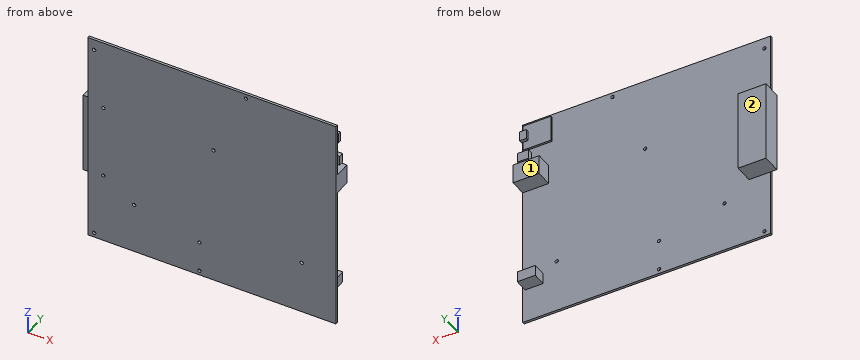
from build123d import *

# Parameters (mm, degrees)
SKETCH1_W               = 203.2
SKETCH1_H               = 177.8
BOSS_EXTRUDE1_DEPTH     = 2
SKETCH3_W               = 21.35
SKETCH3_H               = 16
BOSS_EXTRUDE2_DEPTH     = 13.4
CUT_EXTRUDE1_DEPTH      = 136.666244881
CUT_EXTRUDE1_DEPTH_BACK = 136.666244881
SKETCH2_R               = 1.397
SKETCH4_W               = 22.86
SKETCH4_H               = 67.056
BOSS_EXTRUDE3_DEPTH     = 15.24
SKETCH5_W               = 14.75
SKETCH5_H               = 8.9
BOSS_EXTRUDE4_DEPTH     = 10.922
SKETCH7_W               = 9
SKETCH7_H               = 7.75
BOSS_EXTRUDE5_DEPTH     = 4
SKETCH8_W               = 22.9
SKETCH8_H               = 21.57
BOSS_EXTRUDE6_DEPTH     = 1.6
SKETCH9_W               = 5.5
SKETCH9_H               = 8
BOSS_EXTRUDE7_DEPTH     = 2.7


with BuildPart() as part:
    # Sketch1 → Boss-Extrude1 (new body)
    with BuildSketch(Plane(origin=(0, 0, 0), x_dir=(1, 0, 0), z_dir=(0, 1, 0))):
        Rectangle(SKETCH1_W, SKETCH1_H)
    extrude(amount=BOSS_EXTRUDE1_DEPTH)

    # Sketch3 → Boss-Extrude2 (add)
    with BuildSketch(Plane(origin=(0, 2, 0), x_dir=(1, 0, 0), z_dir=(0, 1, 0))):
        with Locations((90.925, -35.94)):
            Rectangle(SKETCH3_W, SKETCH3_H)
    extrude(amount=BOSS_EXTRUDE2_DEPTH)

    # Sketch2 → Cut-Extrude1 (cut, two sides: drawn at the far end of the back side and taken through both)
    with BuildSketch(Plane(origin=(0, 2, 0), x_dir=(1, 0, 0), z_dir=(0, 1, 0)).offset(-CUT_EXTRUDE1_DEPTH_BACK)):
        with Locations(Location((-96.52, 85.09, 0), (0, 0, 270))):
            Circle(SKETCH2_R)
        with Locations(Location((-10.16, 85.09, 0), (0, 0, 270))):
            Circle(SKETCH2_R)
        with Locations(Location((-10.16, 59.69, 0), (0, 0, 270))):
            Circle(SKETCH2_R)
        with Locations(Location((73.66, 44.831, 0), (0, 0, 270))):
            Circle(SKETCH2_R)
        with Locations(Location((-63.754, 46.99, 0), (0, 0, 270))):
            Circle(SKETCH2_R)
        with Locations(Location((1.27, -27.94, 0), (0, 0, 270))):
            Circle(SKETCH2_R)
        with Locations(Location((-96.52, -79.756, 0), (0, 0, 270))):
            Circle(SKETCH2_R)
        with Locations(Location((27.94, -85.09, 0), (0, 0, 270))):
            Circle(SKETCH2_R)
        with Locations(Location((-88.9, -30.48, 0), (0, 0, 270))):
            Circle(SKETCH2_R)
        with Locations(Location((-88.9, 30.48, 0), (0, 0, 270))):
            Circle(SKETCH2_R)
    extrude(amount=CUT_EXTRUDE1_DEPTH + CUT_EXTRUDE1_DEPTH_BACK, mode=Mode.SUBTRACT)

    # Sketch4 → Boss-Extrude3 (add)
    with BuildSketch(Plane(origin=(0, 2, 0), x_dir=(1, 0, 0), z_dir=(0, 1, 0))):
        with Locations((-95.25, 0)):
            Rectangle(SKETCH4_W, SKETCH4_H)
    extrude(amount=BOSS_EXTRUDE3_DEPTH)

    # Sketch5 → Boss-Extrude4 (add)
    with BuildSketch(Plane(origin=(0, 2, 0), x_dir=(1, 0, 0), z_dir=(0, 1, 0))):
        with Locations((92.225, 55.95)):
            Rectangle(SKETCH5_W, SKETCH5_H)
    extrude(amount=BOSS_EXTRUDE4_DEPTH)

    # Sketch7 → Boss-Extrude5 (add)
    with BuildSketch(Plane(origin=(0, 2, 0), x_dir=(1, 0, 0), z_dir=(0, 1, 0))):
        with Locations((98.95, -57.575)):
            Rectangle(SKETCH7_W, SKETCH7_H)
    extrude(amount=BOSS_EXTRUDE5_DEPTH)

    # Sketch8 → Boss-Extrude6 (add)
    with BuildSketch(Plane(origin=(0, 2, 0), x_dir=(1, 0, 0), z_dir=(0, 1, 0))):
        with Locations((88.9, -75.615)):
            Rectangle(SKETCH8_W, SKETCH8_H)
    extrude(amount=BOSS_EXTRUDE6_DEPTH)

    # Sketch9 → Boss-Extrude7 (add)
    with BuildSketch(Plane(origin=(0, 3.6, 0), x_dir=(1, 0, 0), z_dir=(0, 1, 0))):
        with Locations((98.85, -75.9)):
            Rectangle(SKETCH9_W, SKETCH9_H)
    extrude(amount=BOSS_EXTRUDE7_DEPTH)


solid = part.part
Can you work these out from the model? Positions are in its coordinate system, mm. Face numbers are marked on the shaded views. A direction names the side the tool comes from. Coordinates: 2 decimals unless noted, no trailing zeros. Write each loop counter-clockwise with the first axis right and the second up, starting at its lowest first coordinate (ties: lowest second). Pieces come first, ordered by that corner, then holes.
Q1. Imagine slicing it at D-D, the plane z = -69. List the corners of the cut face in (x, y) for me, plus the area to 3 significant figures.
Results found:
outline: (-101.6, 0) - (101.6, 0) - (101.6, 2) - (-101.6, 2) - close
area: 406 mm2
Q2. Imagine slicing it at B-B, the plane z = 57. List the corners of the cut face in (x, y) for me, plus the area to 3 significant figures.
Results found:
outline: (-101.6, 0) - (101.6, 0) - (101.6, 2) - (103.45, 2) - (103.45, 6) - (94.45, 6) - (94.45, 2) - (-101.6, 2) - close
area: 442 mm2
Q3. Which directions (+Z, -Z, +X, -X, +Y, -Y) give clear straight access to the entire face, cutting with the end or side of a thin tool? Please do the marked faces 1 and 2.
Results found:
face 1: +Z, -Z, +X, +Y
face 2: +Z, -Z, +X, -X, +Y
Q4. Imagine slicing it at A-A, the plane y = 9.75. List the corners of the cut face in (x, z) for me, plus the area to 3 significant figures.
Results found:
outline: (-106.68, -33.53) - (-83.82, -33.53) - (-83.82, 33.53) - (-106.68, 33.53) - close; (80.25, 27.94) - (101.6, 27.94) - (101.6, 43.94) - (80.25, 43.94) - close; (84.85, -60.4) - (99.6, -60.4) - (99.6, -51.5) - (84.85, -51.5) - close
area: 2,010 mm2
Q5. Imagine slicing it at C-C, the plane z = 13. List the corners of the cut face in (x, y) for me.
Results found:
outline: (-106.68, 2) - (-101.6, 2) - (-101.6, 0) - (101.6, 0) - (101.6, 2) - (-83.82, 2) - (-83.82, 17.24) - (-106.68, 17.24) - close
Q6. For P1, Ø0.8, axis at y = 2.5, z = 77.5, coming from the -X side; P2, Ø3, axis at x = 97, y = 5, coming from the +Z side; P3, Ø1, axis at y = 1, z = 1, coming from the -X side; P4, Ø2, axis at x = 22, y = 4, coming from the +Z side, each with a flat end and sliding along its axis, tell me the tip position at first contact or that it passes through.
Results found:
P1: stops at x = 77.45
P2: stops at z = 86.4
P3: stops at x = -101.6
P4: passes through
Q7. Please list where these lines run through material, in increasing order: L1, parallel to Z at x = -88.9, y = 0.65; L2, parallel to Z at x = 93.5, y = 2.5; L3, parallel to Z at x = 27.94, y = 1.3.
Results found:
L1: z = -88.9 to -31.88, -29.08 to 29.08, 31.88 to 88.9
L2: z = -60.4 to -51.5, 27.94 to 43.94, 64.83 to 86.4
L3: z = -88.9 to 83.69, 86.49 to 88.9
